```python
from build123d import *

# Parameters (mm, degrees)
F0_W          = 40
F0_H          = 210
F0_R          = 2.2155
F0_W_2        = 10
F0_H_2        = 170
F1_DEPTH      = 2.5
F1_DEPTH_BACK = 2.5
F2_R          = 4.99999


# Not quite as in the source:
# - a fillet or chamfer is up to 0.001 mm smaller than in the source, because OpenCascade refuses the exact size


with BuildPart() as f1:
    # F0 (on Top) → F1 (new body, two sides)
    with BuildSketch(Plane.XY) as f1_sk:
        Rectangle(F0_W, F0_H)
        with Locations((-15, -75)):
            Circle(F0_R, mode=Mode.SUBTRACT)
        with Locations((-15, -35)):
            Circle(F0_R, mode=Mode.SUBTRACT)
        with Locations((15, -75)):
            Circle(F0_R, mode=Mode.SUBTRACT)
        with Locations((15, -35)):
            Circle(F0_R, mode=Mode.SUBTRACT)
        with Locations((-15, 5)):
            Circle(F0_R, mode=Mode.SUBTRACT)
        with Locations((-15, 45)):
            Circle(F0_R, mode=Mode.SUBTRACT)
        with Locations((-15, 85)):
            Circle(F0_R, mode=Mode.SUBTRACT)
        Rectangle(F0_W_2, F0_H_2, mode=Mode.SUBTRACT)
        with Locations((15, 5)):
            Circle(F0_R, mode=Mode.SUBTRACT)
        with Locations((15, 45)):
            Circle(F0_R, mode=Mode.SUBTRACT)
        with Locations((15, 85)):
            Circle(F0_R, mode=Mode.SUBTRACT)
    extrude(amount=F1_DEPTH)
    extrude(f1_sk.sketch, amount=-F1_DEPTH_BACK)

    # F2 (radius 5 in the source; OpenCascade refuses exactly that, so slightly less here)
    f2_edges = [f1.edges().sort_by_distance(p)[0] for p in [
        (-5, 85, 0),
        (5, 85, 0),
        (-5, -85, 0),
        (5, -85, 0),
    ]]
    fillet(f2_edges, radius=F2_R)


solid = f1.part
```
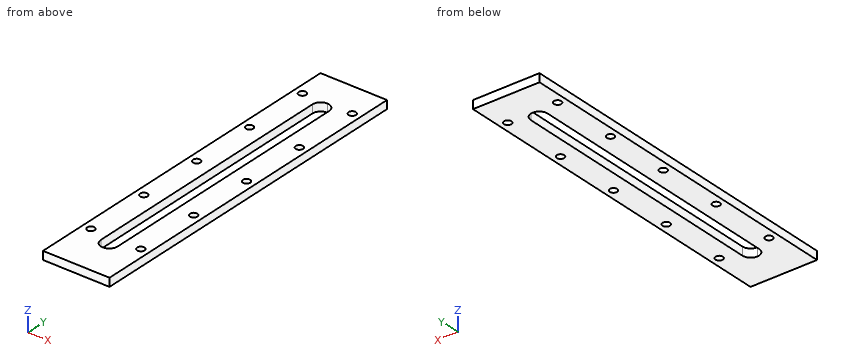
Could you check a few things on this model? Use its own coordinates, in mm. Coordinates: 2 decimals unless noted, no trailing zeros. Write each loop counter-clockwise with the first axis right and the second up, starting at its lowest first coordinate (ties: lowest second). Pieces come first, ordered by that corner, then holes. Notation, with made-up numbers: (84.25, 54.25) -> (93.25, 54.25) arc R30 cw to (93.25, 93.25) -> close; hole circle Ø8 at (65, 34). An arc over 180 degrees is marked (long way). Write item = value, one per line. Start each with the question number.
(1) I want a section at C-C (x = -15). Please give me the cut outline in (y, z).
(2) I want a section at A-A (y = -75). Please give me the cut outline in (x, z).
(3) I want a section at B-B (z = 0.7). Give the number of separate pieces and of enclosed holes in the cut face, plus the area to 3 significant figures.
(4) Will these pins go through, and if not, where does the flat tip stop? pin 1 (3.5 mm diameter, centred on x = -15, y = 5, fed in from -Z); pin 2 (7 mm diameter, centred on x = 15, y = 5, fed in from +Z).
(5) I need wall thicknesses on line 1 (Y direction, x = -15, z = -1.2); line 2 (Y direction, x = -0.5, z = -0.75); line 3 (Y direction, x = 13, z = 2.1). Which ranges of each line are inside material? Lowest first, please. Write a range as [from, to].
Result set:
q1.outline = (-105, -2.5) -> (-77.22, -2.5) -> (-77.22, 2.5) -> (-105, 2.5) -> close; (-72.78, -2.5) -> (-37.22, -2.5) -> (-37.22, 2.5) -> (-72.78, 2.5) -> close; (-32.78, -2.5) -> (2.78, -2.5) -> (2.78, 2.5) -> (-32.78, 2.5) -> close; (7.22, -2.5) -> (42.78, -2.5) -> (42.78, 2.5) -> (7.22, 2.5) -> close; (47.22, -2.5) -> (82.78, -2.5) -> (82.78, 2.5) -> (47.22, 2.5) -> close; (87.22, -2.5) -> (105, -2.5) -> (105, 2.5) -> (87.22, 2.5) -> close
q2.outline = (-20, -2.5) -> (-17.22, -2.5) -> (-17.22, 2.5) -> (-20, 2.5) -> close; (-12.78, -2.5) -> (-5, -2.5) -> (-5, 2.5) -> (-12.78, 2.5) -> close; (5, -2.5) -> (12.78, -2.5) -> (12.78, 2.5) -> (5, 2.5) -> close; (17.22, -2.5) -> (20, -2.5) -> (20, 2.5) -> (17.22, 2.5) -> close
q3.separate_pieces = 1
q3.enclosed_holes = 11
q3.area = 6,570 mm2
q4.pin_1 = through
q4.pin_2 = 2.5
q5.line_1 = [-105, -77.22], [-72.78, -37.22], [-32.78, 2.78], [7.22, 42.78], [47.22, 82.78], [87.22, 105]
q5.line_2 = [-105, -84.97], [84.97, 105]
q5.line_3 = [-105, -75.95], [-74.05, -35.95], [-34.05, 4.05], [5.95, 44.05], [45.95, 84.05], [85.95, 105]
